from build123d import *

# Parameters (mm, degrees)
SKETCH3_W           = 270
SKETCH3_H           = 230
BOSS_EXTRUDE1_DEPTH = 4
SKETCH4_W           = 25
SKETCH4_H           = 70
CUT_EXTRUDE1_DEPTH  = 10
SKETCH6_W           = 25
SKETCH6_H           = 70
CUT_EXTRUDE2_DEPTH  = 10
SKETCH9_R           = 2
CUT_EXTRUDE3_DEPTH  = 10
SKETCH10_R          = 2
CUT_EXTRUDE4_DEPTH  = 10
SKETCH12_R          = 2
CUT_EXTRUDE5_DEPTH  = 10
SKETCH14_R          = 2
CUT_EXTRUDE7_DEPTH  = 10
SKETCH15_R          = 2
CUT_EXTRUDE8_DEPTH  = 10


with BuildPart() as part:
    # Sketch3 → Boss-Extrude1 (new body)
    with BuildSketch(Plane.XY):
        with Locations((0, 115)):
            Rectangle(SKETCH3_W, SKETCH3_H)
    extrude(amount=BOSS_EXTRUDE1_DEPTH)

    # Sketch4 → Cut-Extrude1 (cut)
    with BuildSketch(Plane.XY.offset(4)):
        with Locations((-122.5, 46.430334796)):
            Rectangle(SKETCH4_W, SKETCH4_H)
    extrude(amount=-CUT_EXTRUDE1_DEPTH, mode=Mode.SUBTRACT)

    # Sketch6 → Cut-Extrude2 (cut)
    with BuildSketch(Plane.XY.offset(4)):
        with Locations((122.5, 46.430334796)):
            Rectangle(SKETCH6_W, SKETCH6_H)
    extrude(amount=-CUT_EXTRUDE2_DEPTH, mode=Mode.SUBTRACT)

    # Sketch9 → Cut-Extrude3 (cut)
    with BuildSketch(Plane(origin=(0, 0, 0), x_dir=(-1, 0, 0), z_dir=(0, 0, -1))):
        with Locations((-100, 46.430334796)):
            Circle(SKETCH9_R)
        with Locations((100, 46.186428088)):
            Circle(SKETCH9_R)
    extrude(amount=-CUT_EXTRUDE3_DEPTH, mode=Mode.SUBTRACT)

    # Sketch10 → Cut-Extrude4 (cut)
    with BuildSketch(Plane(origin=(0, 0, 0), x_dir=(-1, 0, 0), z_dir=(0, 0, -1))):
        with Locations((-19.25, 206.268311878)):
            Circle(SKETCH10_R)
        with Locations((19.25, 206.268311878)):
            Circle(SKETCH10_R)
    extrude(amount=-CUT_EXTRUDE4_DEPTH, mode=Mode.SUBTRACT)

    # Sketch12 → Cut-Extrude5 (cut)
    with BuildSketch(Plane.XY.offset(4)):
        with Locations((-125, 140)):
            Circle(SKETCH12_R)
        with Locations((125, 140)):
            Circle(SKETCH12_R)
        with Locations((0, 10)):
            Circle(SKETCH12_R)
    extrude(amount=-CUT_EXTRUDE5_DEPTH, mode=Mode.SUBTRACT)

    # Sketch14 → Cut-Extrude7 (cut)
    with BuildSketch(Plane.XY.offset(4)):
        with Locations((0, 165)):
            Circle(SKETCH14_R)
    extrude(amount=-CUT_EXTRUDE7_DEPTH, mode=Mode.SUBTRACT)

    # Sketch15 → Cut-Extrude8 (cut)
    with BuildSketch(Plane.XY.offset(4)):
        with Locations((92, 53.430334796)):
            Circle(SKETCH15_R)
        with Locations((92, 39.430334796)):
            Circle(SKETCH15_R)
    cut_extrude8 = extrude(amount=-CUT_EXTRUDE8_DEPTH, mode=Mode.SUBTRACT)

    # Mirror1: Cut-Extrude8 across plane
    add(cut_extrude8.mirror(Plane(origin=(0, 0, 0), x_dir=(0, 0, 1), z_dir=(1, 0, 0))), mode=Mode.SUBTRACT)


solid = part.part
Input: part model. Units: mm. Frame: model coordinates. Coordinates: 2 decimals unless noted, no trailing zeros. Loops run counter-clockwise (first coordinate to the right, second up) from the corner with the lowest first, then second, coordinate; pieces in that order, holes last. Notation, with made-up numbers: (82.25, -14) -> (116.25, -14) arc R18 ccw to (116.25, 14) -> close; hole circle Ø11 at (8.5, 64). An arc over 180 degrees is marked (long way). Write item = value, one per line. Start each with the question number.
Item 1: Cut plane B-B, the plane y = 28.5. Return loops of the section in (x, z), plus the area to 3 significant figures.
Item 2: Cut plane A-A, the plane z = 1.1. Count the separate pieces of the cut face and the enclosed holes in it, plus the area to 3 significant figures.
Item 3: First-contact query: P1, Ø4, axis at x = 10, y = 81.5, coming from the -Z side; P2, Ø1.2, axis at y = 48.5, z = 2, coming from the -X side; P3, Ø2, axis at y = 29.5, z = 3, coming from the +X side. Flat tips, straight axial feed; report the tip coordinate or a pass-through.
Item 4: Material intervals for line 1 (X direction, y = 140, z = 1.4); line 2 (Y direction, x = -92, z = 1.3); line 3 (Y direction, x = 0, z = 2.9), sorted ascending.
Ans:
q1.outline = (-110, 0) -> (110, 0) -> (110, 4) -> (-110, 4) -> close
q1.area = 880 mm²
q2.separate_pieces = 1
q2.enclosed_holes = 12
q2.area = 58,400 mm²
q3.P1 = 0
q3.P2 = -110
q3.P3 = 110
q4.line_1 = -135 to -127, -123 to 123, 127 to 135
q4.line_2 = 0 to 37.43, 41.43 to 51.43, 55.43 to 230
q4.line_3 = 0 to 8, 12 to 163, 167 to 230
